Could you check a few things on this drawing? It's one solid part, dimensions in mm from its lowest x, y, z. A direction names the side the tool comes from. Coordinates: 2 decimals unless noted, no trailing zeros. Loops run counter-clockwise (first coordinate to the right, second up) from the corner with the lowest first, then second, coordinate; pieces in that order, holes last.
1) Imagine slicing it at A-A on y = 20. Please give me the cut outline in (x, z).
2) Thinking about a two-plate mould opening in Z: for the marked faces 1, 2, 3 and 4, which applies, released by +Z, released by -Z, zero draft, split by the parting line, or undercut?
3) Will these pins go through, and if not, where does the flat tip stop? P1, Ø11, axis at x = 30, y = 20, coming from the -Z side; P2, Ø1, axis at y = 6.5, z = 31.5, coming from the +X side.
4) If I drill on line 1 along Z through (x, y) = (40.5, 11); line 2 along X through (y, z) = (20, 11); line 3 along Y through (x, z) = (30, 49), over which ranges is the centre line in solid material (lowest first)?
5) Imagine slicing it at C-C on x = 30. Please give me the cut outline in (y, z).
6) Imagine slicing it at D-D on x = 38.5. Please give me the cut outline in (y, z), plus the area to 3 significant figures.
7) For the marked faces 5 and 6, which set-ups out of +Z, -Z, +X, -X, +Y, -Y let a thin tool reach every point of the face, with its end or its side?
8) Imagine slicing it at B-B on z = 28. Please give me the cut outline in (x, y).
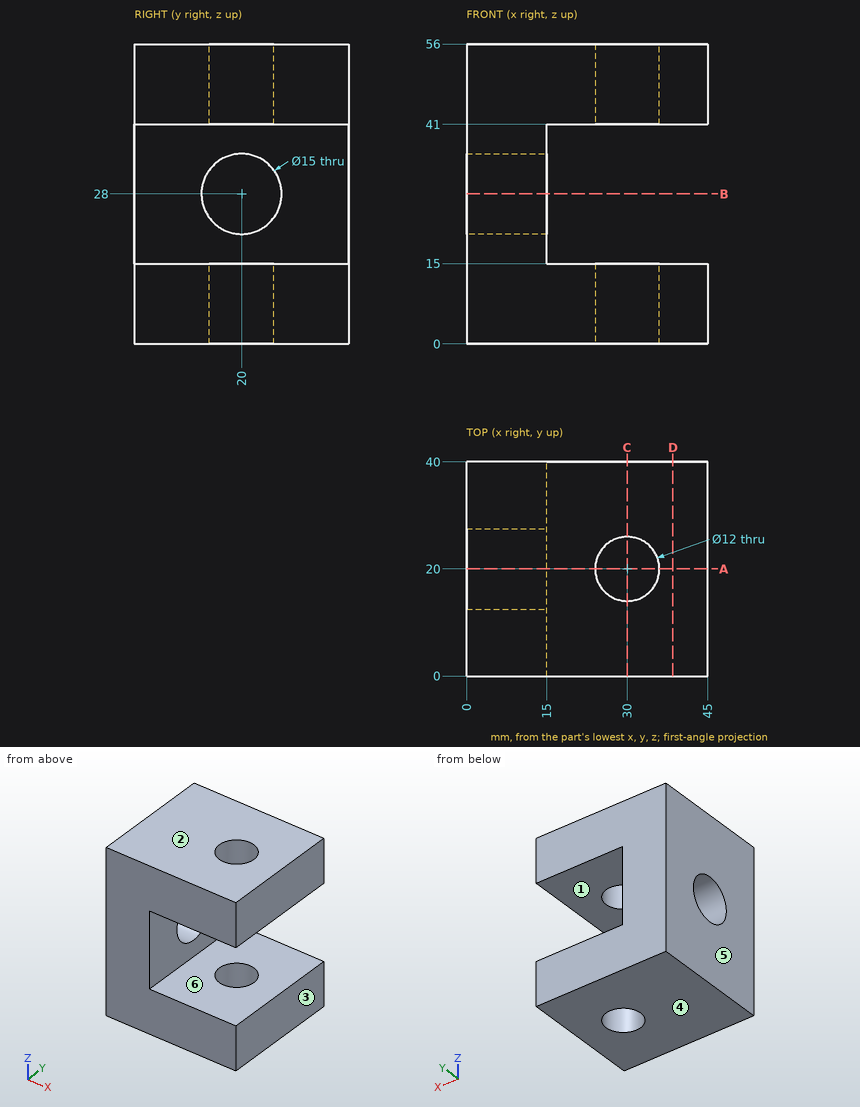
Filled in:
1. outline: (0, 0) - (24, 0) - (24, 15) - (15, 15) - (15, 20.5) - (0, 20.5) - close; (0, 35.5) - (15, 35.5) - (15, 41) - (24, 41) - (24, 56) - (0, 56) - close; (36, 0) - (45, 0) - (45, 15) - (36, 15) - close; (36, 41) - (45, 41) - (45, 56) - (36, 56) - close
2. face 1: undercut
2. face 2: released by +Z
2. face 3: zero draft
2. face 4: released by -Z
3. P1: passes through
3. P2: stops at x = 15
4. line 1: z = 0 to 15, 41 to 56
4. line 2: x = 0 to 24, 36 to 45
4. line 3: y = 0 to 14, 26 to 40
5. outline: (0, 0) - (14, 0) - (14, 15) - (0, 15) - close; (0, 41) - (14, 41) - (14, 56) - (0, 56) - close; (26, 0) - (40, 0) - (40, 15) - (26, 15) - close; (26, 41) - (40, 41) - (40, 56) - (26, 56) - close
6. outline: (0, 0) - (40, 0) - (40, 15) - (0, 15) - close; (0, 41) - (40, 41) - (40, 56) - (0, 56) - close
6. area: 1,200 mm2
7. face 5: +Z, -Z, -X, +Y, -Y
7. face 6: +X, +Y, -Y
8. outline: (0, 0) - (15, 0) - (15, 12.5) - (0, 12.5) - close; (0, 27.5) - (15, 27.5) - (15, 40) - (0, 40) - close
